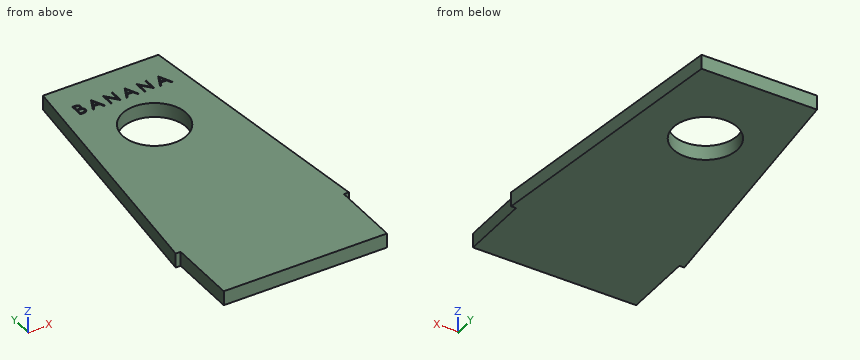
from build123d import *

# Parameters (mm, degrees)
SKETCH1_R           = 5.25
BOSS_EXTRUDE1_DEPTH = 5
SKETCH3_R           = 11.1
CUT_EXTRUDE1_DEPTH  = 6
WRAP1_START         = -4
WRAP1_DEPTH         = 4
SKETCH5_W           = 56.56
SKETCH5_H           = 5
BOSS_EXTRUDE2_DEPTH = 24


# Read off the part's stored shape, not the designer's step: Wrap1
with BuildPart() as part:
    # Sketch1 → Boss-Extrude1 (new body)
    with BuildSketch(Plane.XY):
        Polygon((-30, 0), (30, 0), (20, 90), (-20, 90), align=None)
        with Locations((0, 60)):
            Circle(SKETCH1_R, mode=Mode.SUBTRACT)
    extrude(amount=BOSS_EXTRUDE1_DEPTH)

    # Sketch3 → Cut-Extrude1 (cut)
    with BuildSketch(Plane.XY.offset(5)):
        with Locations((0, 60)):
            Circle(SKETCH3_R)
    extrude(amount=-CUT_EXTRUDE1_DEPTH, mode=Mode.SUBTRACT)

    # Wrap1 outline → Wrap1 (cut)
    # profile 1 of 6: a face of its own
    with BuildSketch(Plane.XY.offset(5).offset(WRAP1_START)):
        with BuildLine():
            add(Edge.make_bspline(
                [(-14.900841346, 80.5), (-14.857861874, 80.499774035), (-14.774556961, 80.499336059), (-14.653417679, 80.492543462), (-14.539954922, 80.483281601), (-14.434135786, 80.468585767), (-14.336009169, 80.450853482), (-14.245279349, 80.429379719), (-14.162234842, 80.403631216), (-14.063089895, 80.362685997), (-13.950049046, 80.301841923), (-13.827651112, 80.211933768), (-13.722988519, 80.101963458), (-13.632748968, 79.97791433), (-13.561004671, 79.841454052), (-13.509101289, 79.695835095), (-13.476241164, 79.542935713), (-13.472861748, 79.437965912), (-13.471153846, 79.384915865)],
                knots=[0, 0, 0, 0, 0.062594097, 0.121322939, 0.176680142, 0.228365096, 0.276868446, 0.321879128, 0.364098625, 0.403355696, 0.477967948, 0.550535461, 0.623584457, 0.698174882, 0.77335367, 0.847281125, 0.92281834, 1, 1, 1, 1], degree=3))
            Line((-14.900841346, 80.5), (-15.778846154, 80.5))
            Line((-15.778846154, 80.5), (-15.778846154, 76))
            Line((-15.778846154, 76), (-14.561899038, 76))
            add(Edge.make_bspline(
                [(-13.125, 77.27734375), (-13.126255945, 77.233414914), (-13.128727052, 77.1469837), (-13.146958444, 77.020012812), (-13.177827296, 76.898673595), (-13.220347341, 76.782181218), (-13.275841746, 76.670761045), (-13.3433777, 76.564286848), (-13.423903996, 76.463828423), (-13.513984827, 76.368269479), (-13.6158933, 76.282348038), (-13.725842128, 76.205827844), (-13.845215968, 76.142897193), (-13.972054246, 76.090033736), (-14.107779795, 76.049653053), (-14.251783147, 76.021402601), (-14.403940107, 76.002367553), (-14.508352644, 76.000802575), (-14.561899038, 76)],
                knots=[0, 0, 0, 0, 0.061160277, 0.120334558, 0.178180255, 0.235235126, 0.292682961, 0.351186248, 0.41045661, 0.471719854, 0.533761203, 0.595739024, 0.657887515, 0.72129518, 0.786822515, 0.854686154, 0.925477986, 1, 1, 1, 1], degree=3))
            add(Edge.make_bspline(
                [(-13.991286058, 78.427584135), (-13.940165508, 78.407957707), (-13.842359233, 78.37040749), (-13.707762931, 78.304019037), (-13.59179813, 78.231810609), (-13.493573228, 78.152955373), (-13.409567672, 78.067958331), (-13.33621389, 77.975573184), (-13.273623552, 77.874594781), (-13.21999265, 77.76607595), (-13.178144249, 77.651124776), (-13.146803801, 77.530819492), (-13.128845652, 77.405591493), (-13.126290113, 77.320367434), (-13.125, 77.27734375)],
                knots=[0, 0, 0, 0, 0.106057493, 0.202914257, 0.290300165, 0.370222566, 0.446383721, 0.5213969, 0.598291083, 0.676142469, 0.7555287, 0.834887172, 0.916646049, 1, 1, 1, 1], degree=3))
            add(Edge.make_bspline(
                [(-13.471153846, 79.384915865), (-13.472559413, 79.335219722), (-13.475321484, 79.237562115), (-13.501733603, 79.094726831), (-13.543083034, 78.958760979), (-13.600561211, 78.830160769), (-13.675263778, 78.711831838), (-13.763795902, 78.602819638), (-13.870608933, 78.507739708), (-13.950635956, 78.454584548), (-13.991286058, 78.427584135)],
                knots=[0, 0, 0, 0, 0.130569107, 0.256580609, 0.380551617, 0.503622917, 0.625739323, 0.747548582, 0.871766119, 1, 1, 1, 1], degree=3))
        make_face()
        with BuildLine():
            add(Edge.make_bspline(
                [(-14.799879808, 76.461538462), (-14.758712617, 76.462031851), (-14.679368285, 76.462982794), (-14.56480956, 76.466087222), (-14.458631284, 76.473148719), (-14.361317967, 76.484264811), (-14.271818813, 76.496322817), (-14.191207481, 76.512537321), (-14.118830518, 76.531114556), (-14.034906408, 76.559829921), (-13.940401897, 76.604439669), (-13.838559368, 76.671700817), (-13.748011373, 76.751830784), (-13.671118897, 76.844570531), (-13.608102197, 76.945410809), (-13.562259469, 77.052311973), (-13.533985511, 77.163507651), (-13.530562721, 77.239321996), (-13.528846154, 77.27734375)],
                knots=[0, 0, 0, 0, 0.072502489, 0.139738989, 0.201795135, 0.259821934, 0.312205989, 0.360773434, 0.404540343, 0.443698099, 0.516840794, 0.587874336, 0.657965418, 0.728969389, 0.79930772, 0.866635778, 0.933116329, 1, 1, 1, 1], degree=3))
            Line((-14.799879808, 76.461538462), (-15.375, 76.461538462))
            Line((-15.375, 76.461538462), (-15.375, 78.134615385))
            Line((-15.375, 78.134615385), (-15.107271635, 78.134615385))
            add(Edge.make_bspline(
                [(-14.265324519, 78.081430288), (-14.287219071, 78.085872539), (-14.334690975, 78.095504255), (-14.412100722, 78.105671303), (-14.50047541, 78.114729237), (-14.60001911, 78.121429297), (-14.710857762, 78.128354852), (-14.833228087, 78.131048194), (-14.966630348, 78.134261528), (-15.05919197, 78.134494415), (-15.107271635, 78.134615385)],
                knots=[0, 0, 0, 0, 0.079306486, 0.171952819, 0.277056507, 0.394730576, 0.526177321, 0.671344767, 0.829285257, 1, 1, 1, 1], degree=3))
            add(Edge.make_bspline(
                [(-13.528846154, 77.27734375), (-13.529201145, 77.301120902), (-13.529905402, 77.348291679), (-13.540526192, 77.417612018), (-13.555972596, 77.484759569), (-13.575941583, 77.549916664), (-13.605023755, 77.611905291), (-13.638975027, 77.671951439), (-13.678782543, 77.730134484), (-13.740810757, 77.803693095), (-13.831031879, 77.88844354), (-13.959226305, 77.971420329), (-14.104990688, 78.038338938), (-14.21071175, 78.066752551), (-14.265324519, 78.081430288)],
                knots=[0, 0, 0, 0, 0.060287398, 0.119602355, 0.177503371, 0.235142664, 0.292132593, 0.350871209, 0.410097863, 0.470731522, 0.594828704, 0.722578824, 0.85669139, 1, 1, 1, 1], degree=3))
        make_face(mode=Mode.SUBTRACT)
        with BuildLine():
            add(Edge.make_bspline(
                [(-15.103665865, 78.596153846), (-15.064003128, 78.596668033), (-14.987366638, 78.597661546), (-14.876383914, 78.600507497), (-14.773366033, 78.60847641), (-14.678490819, 78.616443033), (-14.591907677, 78.629396074), (-14.513808427, 78.644814518), (-14.442967373, 78.66112111), (-14.361273672, 78.688853307), (-14.268608453, 78.72983889), (-14.169823033, 78.793445536), (-14.082735858, 78.869205419), (-14.009196616, 78.95662237), (-13.94901044, 79.052878894), (-13.907207092, 79.156439169), (-13.878860584, 79.264722196), (-13.876300043, 79.33905995), (-13.875, 79.376802885)],
                knots=[0, 0, 0, 0, 0.072301034, 0.139700332, 0.202288511, 0.260599533, 0.313190329, 0.361738933, 0.405706476, 0.445539985, 0.518831956, 0.58977824, 0.658867479, 0.728430478, 0.797282704, 0.864815377, 0.931363753, 1, 1, 1, 1], degree=3))
            Line((-15.103665865, 78.596153846), (-15.375, 78.596153846))
            Line((-15.375, 78.596153846), (-15.375, 80.038461538))
            Line((-15.375, 80.038461538), (-14.826923077, 80.038461538))
            add(Edge.make_bspline(
                [(-13.875, 79.376802885), (-13.875676517, 79.401778877), (-13.87700358, 79.450772012), (-13.887872112, 79.52219261), (-13.906344708, 79.589363149), (-13.930071656, 79.653204148), (-13.963228542, 79.711719384), (-14.00226728, 79.766932064), (-14.049434596, 79.816961931), (-14.10312257, 79.863722715), (-14.164847942, 79.905179965), (-14.234573889, 79.941489517), (-14.313243759, 79.970727659), (-14.399531715, 79.99633414), (-14.494765971, 80.01431909), (-14.59784754, 80.029302017), (-14.70962075, 80.036929828), (-14.786950167, 80.03793958), (-14.826923077, 80.038461538)],
                knots=[0, 0, 0, 0, 0.057003133, 0.111817869, 0.164402372, 0.215869805, 0.26684111, 0.317478963, 0.369902136, 0.423400449, 0.479718398, 0.539241497, 0.602430689, 0.671029546, 0.744484798, 0.823453971, 0.908740313, 1, 1, 1, 1], degree=3))
        make_face(mode=Mode.SUBTRACT)
    # profile 2 of 6: a face of its own
    with BuildSketch(Plane.XY.offset(5).offset(WRAP1_START)):
        Polygon((15.685997596, 76), (16.125, 76), (14.048076923, 80.5), (13.990384615, 80.5), (11.855769231, 76), (12.296574519, 76), (12.980769231, 77.442307692), (15.020733173, 77.442307692), align=None)
        Polygon((14.807992788, 77.903846154), (13.199819712, 77.903846154), (14.014723558, 79.622896635), align=None, mode=Mode.SUBTRACT)
    # profile 3 of 6: a face of its own
    with BuildSketch(Plane.XY.offset(5).offset(WRAP1_START)):
        Polygon((9.813822115, 76), (9.905769231, 76), (9.905769231, 80.5), (9.501923077, 80.5), (9.501923077, 76.958233173), (6.528966346, 80.5), (6.444230769, 80.5), (6.444230769, 76), (6.848076923, 76), (6.848076923, 79.533653846), align=None)
    # profile 4 of 6: a face of its own
    with BuildSketch(Plane.XY.offset(5).offset(WRAP1_START)):
        Polygon((4.055228365, 76), (4.494230769, 76), (2.417307692, 80.5), (2.359615385, 80.5), (0.225, 76), (0.665805288, 76), (1.35, 77.442307692), (3.389963942, 77.442307692), align=None)
        Polygon((3.177223558, 77.903846154), (1.569050481, 77.903846154), (2.383954327, 79.622896635), align=None, mode=Mode.SUBTRACT)
    # profile 5 of 6: a face of its own
    with BuildSketch(Plane.XY.offset(5).offset(WRAP1_START)):
        Polygon((-1.816947115, 76), (-1.725, 76), (-1.725, 80.5), (-2.128846154, 80.5), (-2.128846154, 76.958233173), (-5.101802885, 80.5), (-5.186538462, 80.5), (-5.186538462, 76), (-4.782692308, 76), (-4.782692308, 79.533653846), align=None)
    # profile 6 of 6: a face of its own
    with BuildSketch(Plane.XY.offset(5).offset(WRAP1_START)):
        Polygon((-7.575540865, 76), (-7.136538462, 76), (-9.213461538, 80.5), (-9.271153846, 80.5), (-11.405769231, 76), (-10.964963942, 76), (-10.280769231, 77.442307692), (-8.240805288, 77.442307692), align=None)
        Polygon((-8.453545673, 77.903846154), (-10.06171875, 77.903846154), (-9.246814904, 79.622896635), align=None, mode=Mode.SUBTRACT)
    extrude(amount=WRAP1_DEPTH, mode=Mode.SUBTRACT)

    # Sketch5 → Boss-Extrude2 (add)
    with BuildSketch(Plane.XZ):
        with Locations((0, 2.5)):
            Rectangle(SKETCH5_W, SKETCH5_H)
    extrude(amount=BOSS_EXTRUDE2_DEPTH)


solid = part.part
Source: CAD feature listing. Evaluate the final solid. Frame: model axes, mm. Coordinates: 2 decimals unless noted, no trailing zeros. Loops run counter-clockwise (first coordinate to the right, second up) from the corner with the lowest first, then second, coordinate; pieces in that order, holes last. Notation, with made-up numbers: (53.25, -8.75) -> (59.25, -8.75) arc R28 cw to (59.25, 9.25) -> close; hole circle Ø8 at (-27.5, -11). An arc over 180 degrees is marked (long way). Answer in a Markdown table with one row per item. Add a question column.
Q1. Section C-C on x = -3.5. Return the cut outline in (y, z), and give its area (3 significant figures).
Q2. Section D-D on x = -22.5. Return the cut outline in (y, z), and give its area (4 significant figures).
Q3. Section A-A on y = 60. Return the cut outline in (x, z), and give its area (3 significant figures).
Q4. Ray query, line 1 along Y through (x, z) = (0, 3.6); line 2 along X through (y, z) = (61.5, 2.15); line 3 along X through (y, z) = (59.5, 3.2). Return the intervals inside material, ascending.
Q5. Section B-B on z = 2.65. Give the number of separate pieces and of enclosed holes in the cut face, and give its area (3 significant figures).
Q6. Contact query for flat-ended pins moving along their axis: pin 1 Ø3 at (y, z) = (14.5, 1) entering from -X; pin 2 Ø2 at (y, z) = (77, 2) entering from -X; pin 3 Ø1.2 at (y, z) = (78.5, 3) entering from -X. Output: stop coordinate, or through.
Computed values:
| question | item | result |
|---|---|---|
| 1 | outline | (-24, 0) -> (49.47, 0) -> (49.47, 5) -> (-24, 5) -> close; (70.53, 0) -> (90, 0) -> (90, 5) -> (78.59, 5) -> (78.59, 1) -> (78.01, 1) -> (78.01, 5) -> (70.53, 5) -> close |
| 1 | area | 462 mm^2 |
| 2 | outline | (-24, 0) -> (67.5, 0) -> (67.5, 5) -> (-24, 5) -> close |
| 2 | area | 457.5 mm^2 |
| 3 | outline | (-23.33, 0) -> (-11.1, 0) -> (-11.1, 5) -> (-23.33, 5) -> close; (11.1, 0) -> (23.33, 0) -> (23.33, 5) -> (11.1, 5) -> close |
| 3 | area | 122 mm^2 |
| 4 | line 1 | y = -24 to 48.9, 71.1 to 90 |
| 4 | line 2 | x = -23.17 to -11, 11 to 23.17 |
| 4 | line 3 | x = -23.39 to -11.09, 11.09 to 23.39 |
| 5 | separate pieces | 6 |
| 5 | enclosed holes | 7 |
| 5 | area | 5,440 mm^2 |
| 6 | pin 1 | stops at x = -28.56 |
| 6 | pin 2 | stops at x = -21.56 |
| 6 | pin 3 | stops at x = -21.34 |
